Work out the finished part from the listing and answer in its coordinate system (mm). Coordinates: 2 decimals unless noted, no trailing zeros. Write each loop counter-clockwise with the first axis right and the second up, starting at its lowest first coordinate (ties: lowest second). Pieces come first, ordered by that corner, then holes. Notation, with made-up numbers: (-18.5, -26) - (21.5, -26) arc R31 cw to (21.5, 10) - close; hole circle Ø11 at (-4.5, 75). An arc over 180 degrees is marked (long way). Use one line per item in the form item = value. Start each with the question number.
Item 1: A cutting plane is placed at C-C (x = -2.45). Write down the section's boundary in (y, z), then the cut area to 3 significant figures.
Item 2: A cutting plane is placed at B-B (z = -8). Write down the section's boundary in (x, y).
Item 3: Given pin 1 (3 mm diameter, centred on x = -3, y = 12.5, fed in from -Z); pin 2 (1.5 mm diameter, centred on x = -3.5, y = -3, fed in from -Z); pin 3 (1 mm diameter, centred on y = -55.5, z = -24, fed in from +X), each flat-ended and moving along its own axis, determine where each tip first touches the part or whether it passes through.
Item 4: Consider probe 1 along Z at (x, y) = (-1.1, -1); probe 2 along Y at (x, z) = (-3.9, 52); probe 3 along Z at (x, y) = (-0.4, 44.5). Determine where each line is inside the solid, lowest interval first.
Item 5: A cutting plane is placed at A-A (y = 0). Write down the section's boundary in (x, z), then the cut area to 3 significant figures.
Item 6: A cutting plane is placed at D-D (z = 39). Write down the section's boundary in (x, y), then the cut area to 3 significant figures.
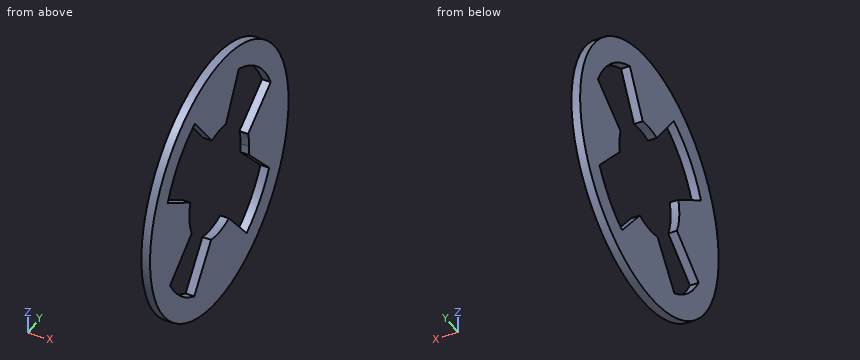
from build123d import *

# Parameters (mm, degrees)
F0_R     = 75.9376
F0_R_2   = 68.52161
F1_DEPTH = 5


with BuildPart() as f1:
    # F0 (on Right) → F1 (new body)
    with BuildSketch(Plane.YZ):
        Circle(F0_R)
        Circle(F0_R_2, mode=Mode.SUBTRACT)
        Circle(F0_R_2)
        with BuildLine():
            ThreePointArc((56.394858, 25.318694), (60.446718, 12.946452), (61.817605, 0))
            ThreePointArc((61.817605, 0), (60.002667, -14.869305), (54.664425, -28.865497))
            ThreePointArc((54.664425, -28.865497), (44.14642, -43.272507), (29.952561, -54.076431))
            ThreePointArc((29.952561, -54.076431), (1.408359, -61.80156), (-27.458115, -55.384729))
            ThreePointArc((-27.458115, -55.384729), (-42.625694, -44.771269), (-53.970641, -30.142764))
            ThreePointArc((-53.970641, -30.142764), (-61.747297, -2.947473), (-56.596401, 24.864908))
            ThreePointArc((-56.596401, 24.864908), (-44.432395, 42.978815), (-26.732948, 55.738369))
            ThreePointArc((-26.732948, 55.738369), (-2.889331, 61.750045), (21.411461, 57.991082))
            ThreePointArc((21.411461, 57.991082), (42.193922, 45.178416), (56.394858, 25.318694))
        make_face(mode=Mode.SUBTRACT)
        with BuildLine():
            Line((-31.792757, 8.234946), (-56.596401, 24.864908))
            ThreePointArc((-56.596401, 24.864908), (-61.747297, -2.947473), (-53.970641, -30.142764))
            Line((-53.970641, -30.142764), (-30.23852, -12.815055))
            ThreePointArc((-30.23852, -12.815055), (-32.752793, -2.418318), (-31.792757, 8.234946))
        make_face()
        with BuildLine():
            Line((7.324043, 32.014874), (21.411461, 57.991082))
            ThreePointArc((21.411461, 57.991082), (-2.889331, 61.750045), (-26.732948, 55.738369))
            Line((-26.732948, 55.738369), (-8.052702, 31.839405))
            ThreePointArc((-8.052702, 31.839405), (-0.374745, 32.839813), (7.324043, 32.014874))
        make_face()
        with BuildLine():
            ThreePointArc((-27.458115, -55.384729), (1.408359, -61.80156), (29.952561, -54.076431))
            Line((29.952561, -54.076431), (10.481953, -31.124306))
            ThreePointArc((10.481953, -31.124306), (0.777417, -32.832748), (-8.997103, -31.585533))
            Line((-8.997103, -31.585533), (-27.458115, -55.384729))
        make_face()
        with BuildLine():
            ThreePointArc((54.664425, -28.865497), (60.002667, -14.869305), (61.817605, 0))
            ThreePointArc((61.817605, 0), (60.446718, 12.946452), (56.394858, 25.318694))
            Line((56.394858, 25.318694), (31.605966, 8.925057))
            ThreePointArc((31.605966, 8.925057), (32.531487, 4.505117), (32.841951, 0))
            ThreePointArc((32.841951, 0), (32.739709, -2.589439), (32.43362, -5.162756))
            Line((32.43362, -5.162756), (54.664425, -28.865497))
        make_face()
    extrude(amount=-F1_DEPTH)


solid = f1.part
Answer:
q1.outline = circle Ø151.88 at (0, 0); hole (-56.6, 24.86) - (-31.79, 8.23) arc R32.84 ccw to (-30.24, -12.82) - (-53.97, -30.14) arc R61.82 ccw to (-27.46, -55.38) - (-9, -31.59) arc R32.84 ccw to (10.48, -31.12) - (29.95, -54.08) arc R61.82 ccw to (54.66, -28.87) - (32.43, -5.16) arc R32.84 ccw to (32.84, 0) arc R32.84 ccw to (31.61, 8.93) - (56.39, 25.32) arc R61.82 ccw to (21.41, 57.99) - (7.32, 32.01) arc R32.84 ccw to (-8.05, 31.84) - (-26.73, 55.74) arc R61.82 ccw to start
q1.area = 10,400 mm²
q2.outline = (-5, -75.52) - (0, -75.52) - (0, -31.85) - (-5, -31.85) - close; (-5, 35.09) - (0, 35.09) - (0, 75.52) - (-5, 75.52) - close
q3.pin_1 = -75.14
q3.pin_2 = -75.9
q3.pin_3 = 0
q4.probe_1 = -75.93 to -32.83, 32.83 to 75.93
q4.probe_2 = -55.34 to -33.43, -23.81 to 18.16, 33.43 to 55.34
q4.probe_3 = -61.53 to -42.91, -18.03 to 17.45, 42.91 to 61.53
q5.outline = (-5, -75.94) - (0, -75.94) - (0, -32.84) - (-5, -32.84) - close; (-5, 32.84) - (0, 32.84) - (0, 75.94) - (-5, 75.94) - close
q5.area = 431 mm²
q6.outline = (-5, -65.16) - (0, -65.16) - (0, -47.96) - (-5, -47.96) - close; (-5, -13.65) - (0, -13.65) - (0, 11.11) - (-5, 11.11) - close; (-5, 47.96) - (0, 47.96) - (0, 65.16) - (-5, 65.16) - close
q6.area = 296 mm²
